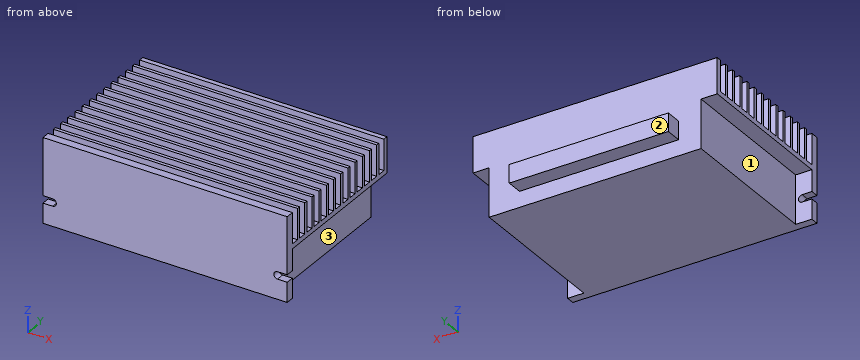
from build123d import *

# Parameters (mm, degrees)
BOSS_EXTRUDE1_DEPTH            = 92
BOSS_EXTRUDE1_DEPTH_BACK       = 5
SKETCH1_W                      = 151
SKETCH1_H                      = 52
CUT_EXTRUDE1_REACH             = 123.821
SKETCH2_W                      = 10
SKETCH2_H                      = 30
CUT_EXTRUDE2_REACH             = 123.821
CUT_EXTRUDE3_REACH             = 123.821
SKETCH4_W                      = 19
SKETCH4_H                      = 5
CUT_EXTRUDE3_DIRECTION_2_REACH = 123.821
LPATTERN1_COUNT                = 13
LPATTERN1_PITCH                = 7
SKETCH5_W                      = 98.406366265
SKETCH5_H                      = 11.254687051
BOSS_EXTRUDE2_DEPTH            = 10


with BuildPart() as part:
    # Sketch1 → Boss-Extrude1 (new, two sides: drawn at the far end of the back side and taken through both)
    with BuildSketch(Plane(origin=(0, 0, 0), x_dir=(1, 0, 0), z_dir=(0, 1, 0)).offset(-BOSS_EXTRUDE1_DEPTH_BACK)):
        Rectangle(SKETCH1_W, SKETCH1_H)
    extrude(amount=BOSS_EXTRUDE1_DEPTH + BOSS_EXTRUDE1_DEPTH_BACK)

    # Sketch2 → Cut-Extrude1 (cut, up to next)
    with BuildSketch(Plane(origin=(0, 0, 0), x_dir=(1, 0, 0), z_dir=(0, 1, 0)), mode=Mode.PRIVATE) as cut_extrude1_sk1:
        with Locations((-70.5, 11)):
            Rectangle(SKETCH2_W, SKETCH2_H)
    cut_extrude1_tool1 = extrude(cut_extrude1_sk1.sketch, amount=CUT_EXTRUDE1_REACH, mode=Mode.PRIVATE) & part.part
    # Sketch2 → Cut-Extrude1 (cut, up to next)
    with BuildSketch(Plane(origin=(0, 0, 0), x_dir=(1, 0, 0), z_dir=(0, 1, 0)), mode=Mode.PRIVATE) as cut_extrude1_sk2:
        with Locations((70.5, 11)):
            Rectangle(SKETCH2_W, SKETCH2_H)
    cut_extrude1_tool2 = extrude(cut_extrude1_sk2.sketch, amount=CUT_EXTRUDE1_REACH, mode=Mode.PRIVATE) & part.part
    add(cut_extrude1_tool1.solids().sort_by_distance((-70.5, 0, -11))[0], mode=Mode.SUBTRACT)
    add(cut_extrude1_tool2.solids().sort_by_distance((70.5, 0, -11))[0], mode=Mode.SUBTRACT)

    # Sketch3 → Cut-Extrude2 (cut, up to next)
    with BuildSketch(Plane(origin=(0, 0, 0), x_dir=(1, 0, 0), z_dir=(0, 1, 0)), mode=Mode.PRIVATE) as cut_extrude2_sk1:
        with BuildLine():
            Line((-69.5, 9.25), (-75.5, 9.25))
            Line((-75.5, 9.25), (-75.5, 13.75))
            Line((-75.5, 13.75), (-69.5, 13.75))
            ThreePointArc((-69.5, 13.75), (-67.25, 11.5), (-69.5, 9.25))
        make_face()
    cut_extrude2_tool1 = extrude(cut_extrude2_sk1.sketch, amount=-CUT_EXTRUDE2_REACH, mode=Mode.PRIVATE) & part.part
    cut_extrude2 = cut_extrude2_tool1.solids().sort_by_distance((-71.600192, 0, -11.5))[0]
    add(cut_extrude2, mode=Mode.SUBTRACT)

    # Mirror1: Cut-Extrude2 across plane
    add(cut_extrude2.mirror(Plane(origin=(0, 0, 0), x_dir=(0, 0, 1), z_dir=(1, 0, 0))), mode=Mode.SUBTRACT)

    # Sketch4 → Cut-Extrude3 (cut, up to next)
    with BuildSketch(Plane(origin=(0, 0, 0), x_dir=(0, 0, -1), z_dir=(1, 0, 0)), mode=Mode.PRIVATE) as cut_extrude3_sk1:
        with Locations((-16.5, 2.5)):
            Rectangle(SKETCH4_W, SKETCH4_H)
    cut_extrude3_tool1 = extrude(cut_extrude3_sk1.sketch, amount=-CUT_EXTRUDE3_REACH, mode=Mode.PRIVATE) & part.part
    cut_extrude3 = cut_extrude3_tool1.solids().sort_by_distance((0, 2.5, 16.5))[0]
    add(cut_extrude3, mode=Mode.SUBTRACT)

    # Sketch4 → Cut-Extrude3 direction 2 (cut, up to next)
    with BuildSketch(Plane(origin=(0, 0, 0), x_dir=(0, 0, -1), z_dir=(1, 0, 0)), mode=Mode.PRIVATE) as cut_extrude3_direction_2_sk1:
        with Locations((-16.5, 2.5)):
            Rectangle(SKETCH4_W, SKETCH4_H)
    cut_extrude3_direction_2_tool1 = extrude(cut_extrude3_direction_2_sk1.sketch, amount=CUT_EXTRUDE3_DIRECTION_2_REACH, mode=Mode.PRIVATE) & part.part
    cut_extrude3_direction_2 = cut_extrude3_direction_2_tool1.solids().sort_by_distance((0, 2.5, 16.5))[0]
    add(cut_extrude3_direction_2, mode=Mode.SUBTRACT)

    # LPattern1: Cut-Extrude3, Cut-Extrude3 direction 2 ×13
    with Locations(*[(0, i * LPATTERN1_PITCH, 0) for i in range(1, LPATTERN1_COUNT)]):
        add(cut_extrude3, mode=Mode.SUBTRACT)
        add(cut_extrude3_direction_2, mode=Mode.SUBTRACT)

    # Sketch5 → Boss-Extrude2 (add)
    with BuildSketch(Plane(origin=(0, 92, 0), x_dir=(1, 0, 0), z_dir=(0, 1, 0))):
        with Locations((-2.452944614, 10.629426659)):
            Rectangle(SKETCH5_W, SKETCH5_H)
    extrude(amount=BOSS_EXTRUDE2_DEPTH)


solid = part.part
CAD build for the part. Positions are in the model's coordinates, mm. Face numbers are marked on the shaded views. A direction names the side the tool comes from. Coordinates: 2 decimals unless noted, no trailing zeros. Write each loop counter-clockwise with the first axis right and the second up, starting at its lowest first coordinate (ties: lowest second). Pieces come first, ordered by that corner, then holes. Notation, with made-up numbers: (79.5, -3) - (127.5, -3) arc R18 cw to (127.5, 27) - close; hole circle Ø10 at (19, 46). An arc over 180 degrees is marked (long way). Use a Markdown table: item, result. Add a question column.
Item 1: Band-saw the part on D-D, the plane z = -11.5. Give the cut face in (x, y).
Item 2: Flat gauge pins, fed straight in: pin 1 (3 mm diameter, centred on x = -41.5, z = 2, fed in from +Y); pin 2 (8 mm diameter, centred on x = 70.5, y = 42, fed in from -Z); pin 3 (1.5 mm diameter, centred on x = -34, y = 51, fed in from +Z). Where does each tip first touch, or does it go through?
Item 3: Drill centre lines: L1, parallel to X at y = 57.5, z = -14.5; L2, parallel to Z at x = 50.5, y = 79.5; L3, parallel to Y at x = -42, z = -1. Where is each one in solid material? Low to high. Write a range as from..to.
Item 4: Band-saw the part on A-A, the plane z = -3. Give the cut face in (x, y).
Item 5: 3-axis set-ups, long thin cutter, end or side, ignore diameter. For the marked faces 1, 2 and 3: which of +Z, -Z, +X, -X, +Y, -Y reach the whole face in a straight line?
Item 6: Band-saw the part on B-B, the plane z = 12. Give the number of separate pieces and of enclosed holes in the cut face, and give its area (3 significant figures).
Item 7: Band-saw the part on C-C, the plane y = 59. Give the cut face in (x, z), and give its area (3 significant figures).
Numbers:
| question | item | result |
|---|---|---|
| 1 | outline | (-67.25, -5) - (67.25, -5) - (67.25, 0) - (65.5, 0) - (65.5, 92) - (46.75, 92) - (46.75, 102) - (-51.66, 102) - (-51.66, 92) - (-65.5, 92) - (-65.5, 0) - (-67.25, 0) - close |
| 2 | pin 1 | y = 92 |
| 2 | pin 2 | z = 4 |
| 2 | pin 3 | z = 7 |
| 3 | L1 | -65.5..65.5 |
| 3 | L2 | -26..7 |
| 3 | L3 | -5..92 |
| 4 | outline | (-75.5, -5) - (75.5, -5) - (75.5, 0) - (65.5, 0) - (65.5, 92) - (-65.5, 92) - (-65.5, 0) - (-75.5, 0) - close |
| 5 | face 1 | -Z, -X, +Y |
| 5 | face 2 | +Z, -Z, +X, -X, +Y |
| 5 | face 3 | -Z, +X, +Y |
| 6 | separate pieces | 14 |
| 6 | enclosed holes | 0 |
| 6 | area | 4,830 mm2 |
| 7 | outline | (-75.5, 4) - (-65.5, 4) - (-65.5, -26) - (65.5, -26) - (65.5, 4) - (75.5, 4) - (75.5, 7) - (-75.5, 7) - close |
| 7 | area | 4,380 mm2 |
